```python
from build123d import *

# Parameters (mm, degrees)
F1_DEPTH     = 12.7
F3_R         = 7.826189497
F3_R_2       = 7.6449247614
F3_R_3       = 9.3914167861
F3_R_4       = 7.5169302634
F2_R         = 6.8354514468
F2_R_2       = 6.4833469735
F2_R_3       = 6.4699307045
F2_R_4       = 6.483339071
F4_DEPTH     = 25.4
F5_W         = 12.7
F5_H         = 45.72
F7_W         = 12.7
F7_H         = 10.16
F9_R         = 5.08
F10_T1_DEPTH = 102.3282991577
F10_T3_DEPTH = 178.5282991577


# Not quite as in the source:
# - a fillet or chamfer that OpenCascade refuses, or shapes differently, is made with other operations: its cross-section is extruded or revolved along the edge and cut away or added


with BuildPart() as f1:
    # F0 (on Top) → F1 (new body)
    with BuildSketch(Plane.XY):
        Polygon((76.2, 21.421205096), (76.2, 38.1), (-76.2, 38.1), (-76.2, -38.1), (76.2, -38.1), align=None)
    extrude(amount=F1_DEPTH)

    # F3 (on face) + F2 (on face) → F4 (cut)
    with BuildSketch(Plane.XY):
        with Locations((-66.4894506335, 28.616681695)):
            Circle(F3_R)
        with Locations((60.850225389, 29.538076371)):
            Circle(F3_R_2)
        with Locations((62.7190470695, -24.263875559)):
            Circle(F3_R_3)
        with Locations((-67.1401694417, -24.8782932758)):
            Circle(F3_R_4)
    with BuildSketch(Plane.XY.offset(12.7)):
        with Locations((63.5566338897, -26.8813353032)):
            Circle(F2_R)
        with Locations((63.1398707628, 29.3819215149)):
            Circle(F2_R_2)
        with Locations((-68.5578212142, -28.5483933985)):
            Circle(F2_R_3)
        with Locations((-66.0572275519, 29.3819215149)):
            Circle(F2_R_4)
    extrude(amount=-F4_DEPTH, mode=Mode.SUBTRACT)

    # F5 (on Front) → F6 (revolve)
    with BuildSketch(Plane.XZ):
        with Locations((6.35, 35.56)):
            Rectangle(F5_W, F5_H)
    revolve(axis=Axis((0, 0, 35.56), (0, 0, -1)))

    # F7 (on Front) → F8 (revolve, cut)
    with BuildSketch(Plane.XZ):
        with Locations((8.7274818003, 36.8085707384)):
            Rectangle(F7_W, F7_H)
    revolve(axis=Axis((0, 0, 12.7), (0, 0, 1)), mode=Mode.SUBTRACT)

    # F9
    f9_edges = [f1.edges().sort_by_distance(p)[0] for p in [
        (-12.7, 0, 58.42),
        (-12.7, 0, 12.7),
    ]]
    fillet(f9_edges, radius=F9_R)

    # F10: chamfer of 5.08 on 9 edges, made by hand

    # F10_s2 → F10_t1 (cut)
    with BuildSketch(Plane.XZ.offset(-51.1641495789)):
        Polygon((71.12, 12.7), (76.2, 7.62), (76.2, 12.7), align=None)
        Polygon((-71.12, 12.7), (-76.2, 7.62), (-76.2, 12.7), align=None)
    extrude(amount=F10_T1_DEPTH, mode=Mode.SUBTRACT)

    # F10_s4 → F10_t3 (cut)
    with BuildSketch(Plane.YZ.offset(-89.2641495789)):
        Polygon((33.02, 12.7), (38.1, 7.62), (38.1, 12.7), align=None)
        Polygon((-33.02, 12.7), (-38.1, 7.62), (-38.1, 12.7), align=None)
    extrude(amount=F10_T3_DEPTH, mode=Mode.SUBTRACT)

    # F10_s5 → F10_t6 (revolve, cut)
    with BuildSketch(Plane.XZ.offset(28.5483933985)):
        Polygon((-57.0078905097, 12.7), (-62.0878905097, 7.62), (-62.0878905097, 12.7), align=None)
    revolve(axis=Axis((-68.5578212142, -28.5483933985, 12.7), (0, 0, 1)), mode=Mode.SUBTRACT)

    # F10_s7 → F10_t8 (revolve, cut)
    with BuildSketch(Plane.XZ.offset(26.8813353032)):
        Polygon((75.4720853364, 12.7), (70.3920853364, 7.62), (70.3920853364, 12.7), align=None)
    revolve(axis=Axis((63.5566338897, -26.8813353032, 12.7), (0, 0, 1)), mode=Mode.SUBTRACT)

    # F10_s9 → F10_t10 (revolve, cut)
    with BuildSketch(Plane.XZ.offset(-29.3819215149)):
        Polygon((-54.493888481, 12.7), (-59.573888481, 7.62), (-59.573888481, 12.7), align=None)
    revolve(axis=Axis((-66.0572275519, 29.3819215149, 12.7), (0, 0, 1)), mode=Mode.SUBTRACT)

    # F10_s11 → F10_t12 (revolve, cut)
    with BuildSketch(Plane.XZ.offset(-29.3819215149)):
        Polygon((74.7032177363, 12.7), (69.6232177363, 7.62), (69.6232177363, 12.7), align=None)
    revolve(axis=Axis((63.1398707628, 29.3819215149, 12.7), (0, 0, 1)), mode=Mode.SUBTRACT)


solid = f1.part
```
Work out the finished part from the listing and answer in its coordinate system (mm). A direction names the side the tool comes from. Round coordinates to 2 decimals unless told otherwise and drop trailing zeros. Write each loop counter-clockwise with the first axis right and the second up, starting at its lowest first coordinate (ties: lowest second). Pieces come first, ordered by that corner, then holes. Notation, with made-up numbers: (-8, 22.5) -> (21, 22.5) arc R19 ccw to (21, 58.5) -> close; hole circle Ø11 at (28, 58.25). An arc over 180 degrees is marked (long way). Write each question's results on one line, items separated by ' | '.
1) Consider line 1 along Z through (x, y) = (42.5, -27.5); line 2 along X through (y, z) = (-0.5, 49.5); line 3 along Z through (x, y) = (69, 21). Determine where each line is inside the solid, lowest interval first. Write a range as [from, to].
Findings:
line 1: z = [0, 12.7] | line 2: x = [-12.69, 12.69] | line 3: z = [0, 11.36]
2) For a pull along Z with two mould halves and no side action, classify faces 3 (the cylindrical face through (2.27, 0.71, 36.88)), 4 (the flat face through (-1.07, 35.52, 10.2)), 5 (the flat face through (-1, 1, 0)) as +Z half, -Z half, draft (parallel to the pull), parting line (faces both ways), or undercut.
Findings:
face 3: undercut | face 4: +Z half | face 5: -Z half
3) The part is cut by section A-A (x = 0). Write down the section's boundary in (y, z), and give its area (3 significant figures).
Findings:
outline: (-38.1, 0) -> (38.1, 0) -> (38.1, 7.62) -> (33.02, 12.7) -> (17.78, 12.7) arc R5.08 cw to (12.7, 17.78) -> (12.7, 31.73) -> (2.38, 31.73) -> (2.38, 41.89) -> (12.7, 41.89) -> (12.7, 53.34) arc R5.08 ccw to (7.62, 58.42) -> (-7.62, 58.42) arc R5.08 ccw to (-12.7, 53.34) -> (-12.7, 41.89) -> (-2.38, 41.89) -> (-2.38, 31.73) -> (-12.7, 31.73) -> (-12.7, 17.78) arc R5.08 cw to (-17.78, 12.7) -> (-33.02, 12.7) -> (-38.1, 7.62) -> close | area: 1,890 mm²
4) Flat-ended cylindrical pins translate along their axes: pin 1 (6 mm diameter, centred on x = 11.5, y = 22.5, fed in from +Z); pin 2 (10 mm diameter, centred on y = 6.5, z = 40, fed in from -X); pin 3 (10 mm diameter, centred on x = -7, y = -11, fed in from +Z). Find the tip coordinate at first contact, or state that the pin passes through.
Findings:
pin 1: stops at z = 12.7 | pin 2: stops at x = -12.56 | pin 3: stops at z = 58.4
5) The part is cut by section B-B (y = 0). Write down the section's boundary in (x, z).
Findings:
outline: (-76.2, 0) -> (76.2, 0) -> (76.2, 7.62) -> (71.12, 12.7) -> (17.78, 12.7) arc R5.08 cw to (12.7, 17.78) -> (12.7, 31.73) -> (2.38, 31.73) -> (2.38, 41.89) -> (12.7, 41.89) -> (12.7, 53.34) arc R5.08 ccw to (7.62, 58.42) -> (-7.62, 58.42) arc R5.08 ccw to (-12.7, 53.34) -> (-12.7, 41.89) -> (-2.38, 41.89) -> (-2.38, 31.73) -> (-12.7, 31.73) -> (-12.7, 17.78) arc R5.08 cw to (-17.78, 12.7) -> (-71.12, 12.7) -> (-76.2, 7.62) -> close
6) Which of the six approach directions +Z, -Z, +X, -X, +Y, -Y give full straight-line access (tool end or side, diameter ignored) to faces 1 (the cylindrical face through (-2.75, 12.4, 24.85)), 2 (the flat face through (0, 0, 58.42))?
Findings:
face 1: +Z | face 2: +Z, +X, -X, +Y, -Y
